Part model, mm, in its own coordinate system. Round coordinates to 2 decimals unless told otherwise and drop trailing zeros. Loops run counter-clockwise (first coordinate to the right, second up) from the corner with the lowest first, then second, coordinate; pieces in that order, holes last.
(1) Flat gauge pins, fed straight in: pin 1 (1 mm diameter, centred on x = 43.5, z = -38, fed in from +Y); pin 2 (2.5 mm diameter, centred on x = 0, z = -35.56, fed in from -Y); pin 3 (12 mm diameter, centred on x = -18.5, y = 22, fed in from -Z). Where does each tip first touch, or does it go through?
(2) Cut at D-D on x = -66. List the corners of the cut face in (y, z), then the cut area to 3 significant figures.
(3) Cut at B-B on z = 14. List the corners of the cut face in (x, y), then the cut area to 3 significant figures.
(4) Probe probe 1 along Y at (x, z) = (-9.5, -67.5); probe 2 along Y at (x, z) = (-54, 14); probe 3 along Z at (x, y) = (-26, 124.5). List the from-to ranges inside material, lowest first.
(5) Cut at A-A on x = -17. List the corners of the cut face in (y, z).
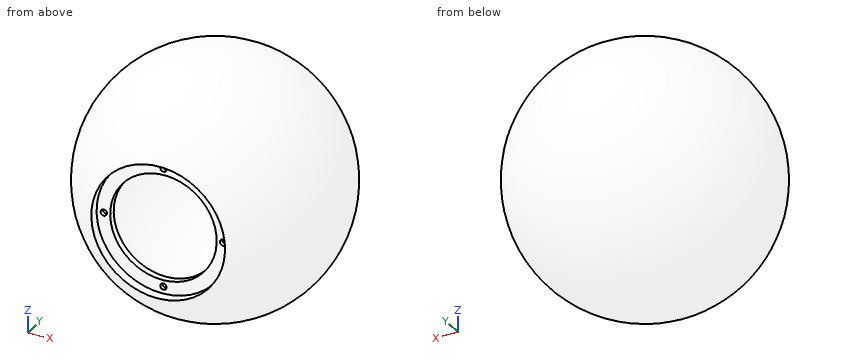
from build123d import *

# Parameters (mm, degrees)
SKETCH2_R          = 1.9
CUT_EXTRUDE1_DEPTH = 2.54


with BuildPart() as part:
    # Sketch1 → Revolve1 (revolve)
    with BuildSketch(Plane(origin=(0, 0, 0), x_dir=(0, 0, -1), z_dir=(1, 0, 0))):
        with BuildLine():
            Line((0, 141.137070307), (0, 139.637070307))
            ThreePointArc((0, 139.637070307), (69.584082777, 92.105902156), (50.616284989, 10))
            Line((50.616284989, 10), (31.75, 10))
            Line((31.75, 10), (31.75, 6))
            Line((31.75, 6), (39.87, 6))
            Line((39.87, 6), (39.87, 0))
            ThreePointArc((39.87, 0), (73.330228274, 85.652224695), (0, 141.137070307))
        make_face()
    revolve(axis=Axis((0, 141.137070307, 0), (0, -1, 0)))

    # Sketch2 → Cut-Extrude1 (cut)
    with BuildSketch(Plane.XZ.offset(-6)):
        with Locations((0, 35.56)):
            Circle(SKETCH2_R)
        with Locations((35.56, 0)):
            Circle(SKETCH2_R)
        with Locations((0, -35.56)):
            Circle(SKETCH2_R)
        with Locations((-35.56, 0)):
            Circle(SKETCH2_R)
    extrude(amount=-CUT_EXTRUDE1_DEPTH, mode=Mode.SUBTRACT)


solid = part.part
Final values:
1. pin 1: stops at y = 115.21
1. pin 2: stops at y = 8.54
1. pin 3: stops at z = -64.39
2. outline: circle Ø76.17 at (64.94, 0); hole circle Ø69.97 at (64.94, 0)
2. area: 711 mm2
3. outline: (-48.64, 10) arc R73.38 cw (long way) to (48.64, 10) - (28.5, 10) - (28.5, 6) - (37.33, 6) - (37.33, 0) arc R74.9 ccw (long way) to (-37.33, 0) - (-37.33, 6) - (-28.5, 6) - (-28.5, 10) - close
3. area: 762 mm2
4. probe 1: y = 30.88 to 34.38, 95.49 to 98.99
4. probe 2: y = 13.03 to 15.26, 114.62 to 116.85
4. probe 3: z = -39.78 to -36.83, 36.83 to 39.78
5. outline: (0, -36.06) arc R74.28 ccw (long way) to (0, 36.06) - (6, 36.06) - (6, 26.82) - (10, 26.82) - (10, 47.68) arc R72.74 cw (long way) to (10, -47.68) - (10, -26.82) - (6, -26.82) - (6, -36.06) - close
